Read the model definition and answer for the solid it produces. Units are mm, in the model's axes. Round coordinates to 2 decimals unless told otherwise and drop trailing zeros. Order: outer loops, then holes, each group sorted by start corner. A loop starts at its lowest first (then second) coordinate and runs counter-clockwise, first axis right, second up. Notation, with made-up numbers: (68.25, -37) - (87.25, -37) arc R31 ccw to (87.25, 1) - close; hole circle Ø11 at (85.25, -20). An arc over 180 degrees is marked (long way). Put each result on its own line as item: value. Start each with the question number.
Q1. Find the intervals of material crossed by line 1 along Y through (x, z) = (4.5, 10.5); line 2 along Y through (x, z) = (0, 20.75); line 3 along Z through (x, y) = (-1, 8), in increasing order. Write a range as from..to.
Q2. Section A-A on y = -17 is taken. Give the vertices of the cut face in (x, z).
Q3. Each of these flat-tipped pins is pushed along its axis until it touches: pin 1 Ø1.5 at (x, z) = (-9.5, 13) entering from +Y; pin 2 Ø5 at (x, y) = (-1, 10) entering from +Z; pin 3 Ø2 at (y, z) = (6, 21) entering from -X. Where does it stop, or does it pass through?
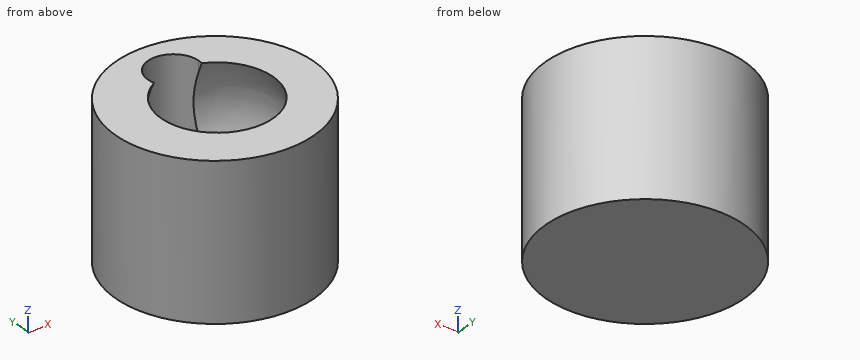
from build123d import *

# Parameters (mm, degrees)
F0_R     = 19.5
F1_DEPTH = 30
F4_R     = 5
F5_DEPTH = 25


with BuildPart() as f1:
    # F0 (on Top) → F1 (new body)
    with BuildSketch(Plane.XY):
        Circle(F0_R)
    extrude(amount=F1_DEPTH)

    # F2 (on Front) → F3 (revolve, cut)
    with BuildSketch(Plane.XZ):
        with BuildLine():
            Line((11.452292, 30), (0.452292, 30))
            Line((0.452292, 30), (0.452292, 5))
            ThreePointArc((0.452292, 5), (11.925941, 14.871595), (11.452292, 30))
        make_face()
    revolve(axis=Axis((0.452292, 0, 17.5), (0, 0, 1)), mode=Mode.SUBTRACT)

    # F4 (on face) → F5 (cut)
    with BuildSketch(Plane.XY.offset(30)):
        with Locations((0, 10.990698)):
            Circle(F4_R)
    extrude(amount=-F5_DEPTH, mode=Mode.SUBTRACT)


solid = f1.part
Findings:
1. line 1: -18.97..-7.72, 7.72..8.81, 13.17..18.97
1. line 2: -19.5..-12.91, 15.99..19.5
1. line 3: 0..5
2. outline: (-9.55, 0) - (9.55, 0) - (9.55, 30) - (-9.55, 30) - close
3. pin 1: y = 17.43
3. pin 2: z = 5
3. pin 3: x = -18.85
